Input: part model. Units: mm. Frame: model coordinates. A direction names the side the tool comes from. Round coordinates to 2 decimals unless told otherwise and drop trailing zeros. Order: outer loops, then holes, each group sorted by start corner. A loop starts at its lowest first (then second) coordinate and runs counter-clockwise, first axis right, second up.
Item 1: Reachability of faces 1 (the flat face through (441.1, 20, 197)), 2 (the flat face through (466, 40, -127)) from +Z, -Z, +X, -X, +Y, -Y: full face, straight path, thin tool, end or side. Return the list, or none.
Item 2: Line query: L1, parallel to X at y = 24.5, z = 260; L2, parallel to Z at x = 466.1, y = 12; L3, parallel to Z at x = 466, y = 11. Output: solid intervals per line, ascending.
Item 3: Cut plane B-B on z = 98. Output: boundary loops of the cut face in (x, y), then the cut area to 3 significant figures.
Item 4: First-contact query: pin 1 (5 mm diameter, centred on y = 29.5, z = 10, fed in from -X). Flat tip, straight axial feed; report the tip coordinate or a pass-through.
Item 5: Cut plane A-A on y = 17. Output: boundary loops of the cut face in (x, z), then the cut area to 3 significant figures.
Autodesk Inventor part; units mm, degrees
ref_plane "YZ Plane" through (0, 0, 0) normal (1, 0, 0) x (0, 1, 0)
ref_plane "XZ Plane" through (0, 0, 0) normal (0, 1, 0) x (-1, 0, 0)
ref_plane "XY Plane" through (0, 0, 0) normal (0, 0, 1) x (1, 0, 0)
sketch "Sketch1" plane through (0, 0, 0) normal (0, 1, 0) x (-1, 0, 0)
  line L0 (0, 329.241) -> (0, -329.241) construction
  line L1 (203.5937, 0) -> (-203.5937, 0) construction
  arc A0 (-441.1, 0) -> (220, -382.3208) centre (0, 0) ccw
  line L2 (-441.1, 0) -> (-441.1, 400)
  line L3 (-441.1, 400) -> (-500, 400)
  line L4 (-500, 400) -> (-500, -500)
  line L5 (-500, -500) -> (220, -500)
  line L6 (220, -500) -> (220, -382.3208)
  dimension "d0" = 500
  dimension "d1" = 400
  dimension "d2" = 500
  dimension "d3" = 441.1
  dimension "d4" = 720
extrude "Extrusion1" add sketch "Sketch1" along normal blind 40
sketch "Sketch3" plane through (0, 0, 0) normal (0, -1, 0) x (1, 0, 0)
  line L0 (500, -472.3208) -> (410, -472.3208)
  line L1 (410, -472.3208) -> (410, 417.6792)
  line L2 (410, 417.6792) -> (500, 417.6792)
  line L3 (500, 417.6792) -> (500, -472.3208)
  line L4 (500, 400) -> (500, -500)
  arc A0 (-220, -382.3208) -> (441.1, 0) centre (0, 0) ccw
  line L5 (441.1, 400) -> (500, 400)
  line L6 (-562.8742, 618.3402) -> (964.0911, 618.3402)
  line L7 (964.0911, 618.3402) -> (964.0911, -811.0554)
  line L8 (964.0911, -811.0554) -> (-562.8742, -811.0554)
  line L9 (-562.8742, -811.0554) -> (-562.8742, 618.3402)
  dimension "d41" = 890
  dimension "d42" = 90
  dimension "d71" = 17.6792
sketch "Sketch4" plane through (0, 0, 0) normal (0, -1, 0) x (1, 0, 0)
  line L0 (441.1, 400) -> (500, 400) construction
  line L1 (441.1, 0) -> (441.1, 400) construction
  arc A0 (-220, -382.3208) -> (441.1, 0) centre (0, 0) ccw construction
  line L2 (464.3817, -39.9852) -> (0, 0) construction
  line L3 (0, 0) -> (445.1648, -138.1214) construction
  line L4 (423.7332, -194.1633) -> (0, 0) construction
  line L5 (360.2723, -295.7246) -> (0, 0) construction
  line L6 (289.0138, -365.6778) -> (0, 0) construction
  line L7 (389.8771, -255.4312) -> (0, 0) construction
  line L8 (326.5218, -332.615) -> (0, 0) construction
  line L9 (230.9911, -404.8361) -> (0, 0) construction
  line L10 (139.32, -444.7911) -> (0, 0) construction
  line L11 (41.2359, -464.2723) -> (0, 0) construction
  line L12 (464.3817, -39.9852) -> (445.1648, -138.1214) construction
  line L13 (445.1648, -138.1214) -> (423.7332, -194.1633) construction
  line L14 (423.7332, -194.1633) -> (389.8771, -255.4312) construction
  line L15 (389.8771, -255.4312) -> (360.2723, -295.7246) construction
  line L16 (360.2723, -295.7246) -> (326.5218, -332.615) construction
  line L17 (326.5218, -332.615) -> (289.0138, -365.6778) construction
  line L18 (289.0138, -365.6778) -> (230.9911, -404.8361) construction
  line L19 (230.9911, -404.8361) -> (139.32, -444.7911) construction
  line L20 (139.32, -444.7911) -> (41.2359, -464.2723) construction
  line L21 (-58.7462, -462.3831) -> (0, 0) construction
  line L22 (-156.0243, -439.2102) -> (0, 0) construction
  line L23 (-200, -421.0098) -> (0, 0) construction
  line L24 (41.2359, -464.2723) -> (-58.7462, -462.3831) construction
  line L25 (-58.7462, -462.3831) -> (-156.0243, -439.2102) construction
  line L26 (-200, -421.0098) -> (-156.0243, -439.2102) construction
  line L27 (-220, -500) -> (-220, -382.3208) construction
  point P0 (466.1, 360)
  point P1 (466.1, 260)
  point P2 (466.1, 160)
  point P3 (466.1, 60)
  dimension "d50" = 40
  dimension "d51" = 100
  dimension "d52" = 100
  dimension "d53" = 100
  dimension "d54" = 25
  dimension "d55" = 466.1
  dimension "d56" = 100
  dimension "d57" = 100
  dimension "d58" = 60
  dimension "d59" = 70
  dimension "d60" = 50
  dimension "d61" = 70
  dimension "d62" = 100
  dimension "d63" = 20
hole "Hole1" at (-200, 0, -421.0098) at (-156.0243, 0, -439.2102) at (-58.7462, 0, -462.3831) at (41.2359, 0, -464.2723) at (139.32, 0, -444.7911) at (230.9911, 0, -404.8361) at (289.0138, 0, -365.6778) at (326.5218, 0, -332.615) at (360.2723, 0, -295.7246) at (389.8771, 0, -255.4312) at (423.7332, 0, -194.1633) at (445.1648, 0, -138.1214) at (464.3817, 0, -39.9852) at (466.1, 0, 60) at (466.1, 0, 160) at (466.1, 0, 260) at (466.1, 0, 360) direction (0, 1, 0) diameter 5.5 end through all
extrude "Extrusion2" cut sketch "Sketch3" against normal through all
fillet "Fillet1" radius 5 2 edges at (500, 20, 400) (500, 20, -472.3208)
properties part number "boundaryV1"
From the geometry:
1. face 1: +Z, -X, +Y, -Y
1. face 2: +Z, -Z, +X, -X, +Y
2. L1: x = 441.1 to 463.35, 468.85 to 500
2. L2: z = -472.32 to -42.13, -37.84 to 57.25, 62.75 to 157.25, 162.75 to 257.25, 262.75 to 357.25, 362.75 to 400
2. L3: z = -472.32 to -42.21, -37.76 to 57.25, 62.75 to 157.25, 162.75 to 257.25, 262.75 to 357.25, 362.75 to 400
3. outline: (441.1, 0) - (500, 0) - (500, 40) - (441.1, 40) - close
3. area: 2,360 mm2
4. pin 1: stops at x = 441.1
5. outline: (410, -472.32) - (495, -472.32) arc R5 ccw to (500, -467.32) - (500, 395) arc R5 ccw to (495, 400) - (441.1, 400) - (441.1, 0) arc R441.1 cw to (410, -162.69) - close; hole circle Ø5.5 at (423.73, -194.16); hole circle Ø5.5 at (445.16, -138.12); hole circle Ø5.5 at (464.38, -39.99); hole circle Ø5.5 at (466.1, 60); hole circle Ø5.5 at (466.1, 160); hole circle Ø5.5 at (466.1, 260); hole circle Ø5.5 at (466.1, 360)
5. area: 62,500 mm2
